Part model, mm, in its own coordinate system. A direction names the side the tool comes from. Give positions to 0.01 mm unless a question says otherwise; leave off trailing zeros. Write each loop counter-clockwise with the first axis right and the second up, starting at its lowest first coordinate (ties: lowest second). Pieces come first, ordered by that corner, then holes. Notation, with made-up numbers: M 39,-26.5 L 88,-26.5 A14 cw 88,-18.5 Z; hole C 22,76.5 d1. An arc over 180 degrees is marked long. Write item = value, one per line. Start each with the question number.
from build123d import *

# Parameters (mm, degrees)
F1_DEPTH = 40
F2_W     = 20
F2_H     = 10
F3_DEPTH = 10
F4_W     = 20
F4_H     = 10
F5_DEPTH = 10


with BuildPart() as f1:
    # F0 (on Front) → F1 (new body)
    with BuildSketch(Plane.XZ):
        Polygon((0, 28.463914), (0, 0), (60, 0), (60, 10), (20, 10), (20, 28.463914), align=None)
    extrude(amount=F1_DEPTH)

    # F2 (on face) → F3 (join)
    with BuildSketch(Plane.XY.offset(10)):
        with Locations((30, -35)):
            Rectangle(F2_W, F2_H)
    extrude(amount=F3_DEPTH)

    # F4 (on face) → F5 (join)
    with BuildSketch(Plane.XY.offset(10)):
        with Locations((30, -5)):
            Rectangle(F4_W, F4_H)
    extrude(amount=F5_DEPTH)


solid = f1.part
Q1. Slice it at D-D (x = 49). Give the cut face in (y, z).
Q2. Drop flat-ended pins along their axis: P1, Ø3, axis at x = 29.5, y = -36.5, coming from the +Z side; P2, Ø15, axis at y = -26, z = 18.5, coming from the +X side; P3, Ø3, axis at y = -33, z = 22, coming from the +X side. Give the stop position or say it passes through.
Q3. Slice it at B-B (x = 29). Give the cut face in (y, z), and give its area (3 significant figures).
Q4. Slice it at A-A (y = -4.5). Give the cut face in (x, z).
Q5. Tool access for faces 4 (the face through (30, -30, 15)), 5 (the face through (10, -20, 28.464)), 6 (the face through (40, -35, 15)): list every direction of +Z, -Z, +X, -X, +Y, -Y with a clear straight run to the whole face (end or side of a thin tool).
Q6. Probe line 1 along Y through (x, z) = (21.5, 13.5); line 2 along X through (y, z) = (-25, 17.25). List the from-to ranges inside material, lowest first.
Q7. Slice it at C-C (y = -12). Give the cut face in (x, z).
Q8. Two-plate mould, pull along Y, no slides. Class faces 1 (the face through (0, -20, 14)), 2 (the face through (23, -40, 11)), 3 (the face through (30, -10, 15)): +Y half, -Y half, draft (parallel to the pull), parting line (faces both ways), or undercut.
Working result:
q1.outline = M -40,0 L 0,0 L 0,10 L -40,10 Z
q2.P1 = 20
q2.P2 = 40
q2.P3 = 20
q3.outline = M -40,0 L 0,0 L 0,20 L -10,20 L -10,10 L -30,10 L -30,20 L -40,20 Z
q3.area = 600 mm2
q4.outline = M 0,0 L 60,0 L 60,10 L 40,10 L 40,20 L 20,20 L 20,28.46 L 0,28.46 Z
q5.face_4 = +Z, +X
q5.face_5 = +Z, +X, -X, +Y, -Y
q5.face_6 = +Z, +X, +Y, -Y
q6.line_1 = -40 to -30, -10 to 0
q6.line_2 = 0 to 20
q7.outline = M 0,0 L 60,0 L 60,10 L 20,10 L 20,28.46 L 0,28.46 Z
q8.face_1 = draft
q8.face_2 = -Y half
q8.face_3 = undercut
